For this review, take the finished solid that the model builds, in its own axes (mm). A direction names the side the tool comes from. Round coordinates to 2 decimals unless told otherwise and drop trailing zeros. Loops run counter-clockwise (first coordinate to the right, second up) from the corner with the lowest first, then second, coordinate; pieces in that order, holes last. Notation, with made-up numbers: M -27,85.5 L 29,85.5 A11 cw 29,101.5 Z; hole C 5.25,37.5 d10. An arc over 180 degrees is marked long. One line per question, with ' | ' between items. Start each with the question number.
1) For faces 4 (the face through (-4.762, -20, 595)), 5 (the face through (0, -18, 0)), list the 3-axis set-ups (+Z, -Z, +X, -X, +Y, -Y) from which the entire face can be reached by the end or side of a thin tool; tool diameter is ignored.
2) We need section B-B (y = 0). Give the boundary of the cut face in (x, z) (3 decimals), and give its area (3 significant figures).
3) Mouldability with a two-part tool opening along Y and no side actions: class faces 1 (the face through (4.762, -20, 595)), 2 (the face through (0, 0, 1219.2)), 3 (the face through (0, -38.1, 595)) as pulls with the +Y half, pulls with the -Y half, needs draft (parallel to the pull), parting line crosses it, or undercut.
4) For probe 1 along X at (y, z) = (-35, 1143) (3 decimals); probe 2 along X at (y, z) = (-33, 990) (3 decimals); probe 3 along X at (y, z) = (-17, 356.5), list the stretches that pass through material, from the lowest coordinate up. Write a range as from..to.
5) For pin 1 Ø15 at (x, y) = (-10, -26.5) entering from +Z; pin 2 Ø2 at (y, z) = (-18, 220) entering from -X; pin 3 Ø10 at (y, z) = (-5, 300.5) entering from +X (3 decimals), all flat-tipped, find the tip position at first contact; note any pin that passes through.
```python
from build123d import *

# Parameters (mm, degrees)
EXTRUDE1_DEPTH         = 1219.2
F_10_CLEARANCE_HOLE1_D = 5.6134
LPATTERN3_COUNT        = 8
LPATTERN3_PITCH        = 152.4
SKETCH4_OUTSIDE_W      = 290.638
SKETCH4_OUTSIDE_H      = 293.813
SKETCH4_OUTSIDE_R      = 9.525
CUT_EXTRUDE1_DEPTH     = 12.7


with BuildPart() as part:
    # Sketch1 → Extrude1 (new body)
    with BuildSketch(Plane.XY):
        with BuildLine():
            Line((-22.225, -38.1), (22.225, -38.1))
            Line((22.225, -38.1), (22.225, -31.75))
            Line((22.225, -31.75), (4.7625, -31.75))
            Line((4.7625, -31.75), (4.7625, -8.248891971))
            ThreePointArc((4.7625, -8.248891971), (0, 9.525), (-4.7625, -8.248891971))
            Line((-4.7625, -8.248891971), (-4.7625, -31.75))
            Line((-4.7625, -31.75), (-22.225, -31.75))
            Line((-22.225, -31.75), (-22.225, -38.1))
        make_face()
    extrude(amount=EXTRUDE1_DEPTH)

    # #10 Clearance Hole1 (through all)
    with Locations(Plane.XZ.offset(38.1)):
        with Locations((-15.875, 76.2), (15.875, 76.2)):
            f_10_clearance_hole1 = Hole(F_10_CLEARANCE_HOLE1_D / 2)

    # LPattern3: #10 Clearance Hole1 ×8
    with Locations(*[(0, 0, i * LPATTERN3_PITCH) for i in range(1, LPATTERN3_COUNT)]):
        add(f_10_clearance_hole1, mode=Mode.SUBTRACT)

    # Sketch4 outside → Cut-Extrude1 (cut)
    with BuildSketch(Plane.XY.offset(1219.2)):
        with Locations((0, -14.2875)):
            Rectangle(SKETCH4_OUTSIDE_W, SKETCH4_OUTSIDE_H)
        with Locations(Location((0, 0, 0), (0, 0, 240))):
            Circle(SKETCH4_OUTSIDE_R, mode=Mode.SUBTRACT)
    extrude(amount=-CUT_EXTRUDE1_DEPTH, mode=Mode.SUBTRACT)


solid = part.part
```
Answers below:
1) face 4: +Z, -Z, -X | face 5: -Z, +X, -X, +Y, -Y
2) outline: M -9.525,0 L 9.525,0 L 9.525,1219.2 L -9.525,1219.2 Z | area: 23,200 mm^2
3) face 1: undercut | face 2: needs draft | face 3: pulls with the -Y half
4) probe 1: -22.225..-18.682, -13.068..13.068, 18.682..22.225 | probe 2: -22.225..-18.617, -13.133..13.133, 18.617..22.225 | probe 3: -4.76..4.76
5) pin 1: z = 1206.5 | pin 2: x = -4.76 | pin 3: x = 9.525
